```python
from build123d import *

# Parameters (mm, degrees)
SKETCH_1_R          = 10
EXTRUDE_1_DEPTH     = 5
EXTRUDE_2_DEPTH     = 5
CUT_EXTRUDE_1_DEPTH = 5
EXTRUDE_3_DEPTH     = 10
SKETCH_5_R          = 1.5
CUT_EXTRUDE_2_DEPTH = 10
SKETCH_6_R          = 1.5
CUT_EXTRUDE_3_DEPTH = 10


with BuildPart() as part:
    # 草图1 → 凸台-拉伸1 (new body)
    with BuildSketch(Plane.XY):
        Circle(SKETCH_1_R)
    extrude(amount=EXTRUDE_1_DEPTH)

    # 草图2 → 凸台-拉伸2 (add)
    with BuildSketch(Plane.XY.offset(5)):
        Polygon((10, 0), (50, 0), (-20.898751954, 36.197700198), (0, 0), align=None)
    extrude(amount=-EXTRUDE_2_DEPTH)

    # 草图3 → 切除-拉伸1 (cut)
    with BuildSketch(Plane.XY.offset(5)):
        Polygon((5.603154877, 25.292377819), (5.603154877, 12.141678981), (11.179717043, 8.31299451), (24.663344965, 16.053595724), align=None)
    extrude(amount=-CUT_EXTRUDE_1_DEPTH, mode=Mode.SUBTRACT)

    # 草图4 → 凸台-拉伸3 (add)
    with BuildSketch(Plane(origin=(0, 0, 0), x_dir=(-1, 0, 0), z_dir=(0, 0, -1))):
        Polygon((-5.603154877, 22.667023681), (-5.603154877, 14.403378326), (6.064261942, 10.503609794), (20.898751954, 36.197700198), align=None)
    extrude(amount=EXTRUDE_3_DEPTH)

    # 草图5 → 切除-拉伸2 (cut)
    with BuildSketch(Plane.XY.offset(5)):
        with Locations((0, 7)):
            Circle(SKETCH_5_R)
        with Locations((7, 0)):
            Circle(SKETCH_5_R)
        with Locations((0, -7)):
            Circle(SKETCH_5_R)
        with Locations((-7, 0)):
            Circle(SKETCH_5_R)
    extrude(amount=-CUT_EXTRUDE_2_DEPTH, mode=Mode.SUBTRACT)

    # 草图6 → 切除-拉伸3 (cut)
    with BuildSketch(Plane.XY.offset(5)):
        Circle(SKETCH_6_R)
    extrude(amount=-CUT_EXTRUDE_3_DEPTH, mode=Mode.SUBTRACT)


solid = part.part
```
The model under review builds one solid part; all positions refer to its coordinate system, in mm. A direction names the side the tool comes from. Give positions to 0.01 mm unless a question says otherwise; leave off trailing zeros. Loops run counter-clockwise (first coordinate to the right, second up) from the corner with the lowest first, then second, coordinate; pieces in that order, holes last. Notation, with made-up numbers: (23.25, 27) - (76.25, 27) arc R22 cw to (76.25, 63) - close; hole circle Ø6 at (73.25, 68). An arc over 180 degrees is marked (long way). Answer as a JSON object with one key per item and string values.
Q1. Add section D-D on y = 7. State the section outline as (x, z) points.
Worked out:
{"outline": "(-7.14, 0) - (-1.5, 0) - (-1.5, 5) - (-7.14, 5) - close; (1.5, 0) - (36.29, 0) - (36.29, 5) - (1.5, 5) - close"}
Q2. Insertion check: pin 1 (4 mm diameter, centred on x = 20.5, z = 2, fed in from -Y); pin 2 (5.5 mm diameter, centred on y = 18.5, z = -1, fed in from +X); pin 3 (4 mm diameter, centred on x = 0, y = 0, fed in from -Z). Each pin has a flat end and moves straight along its axis. Give the tip position at first contact, or say it passes through.
Worked out:
{"pin 1": "stops at y = 0", "pin 2": "stops at x = 5.6", "pin 3": "stops at z = 0"}
Q3. Add section C-C on z = -1. State the section outline as (x, y) points.
Worked out:
{"outline": "(-20.9, 36.2) - (-6.06, 10.5) - (5.6, 14.4) - (5.6, 22.67) - close"}
Q4. Add section A-A on x = 0. State the section outline as (y, z) points, plus the area to 3 significant figures.
Worked out:
{"outline": "(-10, 0) - (-8.5, 0) - (-8.5, 5) - (-10, 5) - close; (-5.5, 0) - (-1.5, 0) - (-1.5, 5) - (-5.5, 5) - close; (1.5, 0) - (5.5, 0) - (5.5, 5) - (1.5, 5) - close; (8.5, 0) - (12.53, 0) - (12.53, -10) - (25.53, -10) - (25.53, 5) - (8.5, 5) - close", "area": "263 mm^2"}
Q5. To check wall thickness, follow line 1 along Y through (x, z) = (-7, 3.8); line 2 along Y through (x, z) = (0, 2.25); line 3 along Z through (x, y) = (31.5, 1). State the ranges of each line that lie inside material, in increasing order.
Worked out:
{"line 1": "y = -7.14 to -1.5, 1.5 to 7.14, 12.12 to 29.1", "line 2": "y = -10 to -8.5, -5.5 to -1.5, 1.5 to 5.5, 8.5 to 25.53", "line 3": "z = 0 to 5"}
Q6. For faces 1 (the flat face through (13, 2, 0)), 2 (the flat face through (-5, 24, -10)), 3 (the flat face through (30, 0, 3)), 4 (the flat face through (8.352, 10.254, 2.535)), 5 (the cylindrical face through (-5.25, -8.51, 2.46)), list the 3-axis set-ups (+Z, -Z, +X, -X, +Y, -Y) from which the entire face can be reached by the end or side of a thin tool; tool diameter is ignored.
Worked out:
{"face 1": "-Z, +X, -Y", "face 2": "-Z, +X, -X, +Y, -Y", "face 3": "+Z, -Z, +X, -Y", "face 4": "+Z, -Z, +Y", "face 5": "+Z, -Z"}
Q7. Mouldability with a two-part tool opening along X and no side actions: class faces 6 (the flat face through (7, 11, 5)), 7 (the flat face through (-0.15, 12.48, -4.93)), 8 (the cylindrical face through (-8.5, 0.07, 2.54)) as +X half, -X half, draft (parallel to the pull), parting line (faces both ways), or undercut.
Worked out:
{"face 6": "draft", "face 7": "+X half", "face 8": "undercut"}
Q8. Add section B-B on y = -7. State the section outline as (x, z) points.
Worked out:
{"outline": "(-7.14, 0) - (-1.5, 0) - (-1.5, 5) - (-7.14, 5) - close; (1.5, 0) - (7.14, 0) - (7.14, 5) - (1.5, 5) - close"}
